from build123d import *

# Parameters (mm, degrees)
SKETCH_1_R          = 6
EXTRUDE_2_DEPTH     = 7.5
CUT_EXTRUDE_START   = -7.5
SKETCH_4_R          = 22.5
CUT_EXTRUDE_4_DEPTH = 2
CUT_EXTRUDE_START_2 = 7.5
SKETCH_4_2_R        = 22.5
CUT_EXTRUDE_5_DEPTH = 2


with BuildPart() as part:
    # 草圖1 → 填料-伸長2 (new body, symmetric)
    with BuildSketch(Plane.XY):
        with BuildLine():
            Line((10.8, 27.988569095), (54.32, 11.195427638))
            ThreePointArc((54.32, 11.195427638), (62, 0), (54.32, -11.195427638))
            Line((54.32, -11.195427638), (10.8, -27.988569095))
            ThreePointArc((10.8, -27.988569095), (2.81349952, -29.867778968), (-5.383437031, -29.513024341))
            ThreePointArc((-5.383437031, -29.513024341), (-23.658051153, -33.253445018), (-34.256327949, -48.603650133))
            ThreePointArc((-34.256327949, -48.603650133), (-47.196522871, -57.898263789), (-57.960436879, -46.151917853))
            ThreePointArc((-57.960436879, -46.151917853), (-46.199430838, -3.114505899), (-13.217722281, 26.931242409))
            ThreePointArc((-13.217722281, 26.931242409), (-1.31940524, 29.97097212), (10.8, 27.988569095))
        make_face()
        with Locations((50, 0)):
            Circle(SKETCH_1_R, mode=Mode.SUBTRACT)
        with Locations((-45.961940777, -45.961940777)):
            Circle(SKETCH_1_R, mode=Mode.SUBTRACT)
        Polygon((15.614971003, -4.18401887), (11.430952133, 11.430952133), (-4.18401887, 15.614971003), (-15.614971003, 4.18401887), (-11.430952133, -11.430952133), (4.18401887, -15.614971003), align=None, mode=Mode.SUBTRACT)
    extrude(amount=EXTRUDE_2_DEPTH, both=True)

    # 草圖4 → 除料-伸長4 (cut)
    with BuildSketch(Plane.XY.offset(CUT_EXTRUDE_START)):
        Circle(SKETCH_4_R)
    extrude(amount=CUT_EXTRUDE_4_DEPTH, mode=Mode.SUBTRACT)

    # 草圖4<2> → 除料-伸長5 (cut)
    with BuildSketch(Plane.XY.offset(CUT_EXTRUDE_START_2)):
        Circle(SKETCH_4_2_R)
    extrude(amount=-CUT_EXTRUDE_5_DEPTH, mode=Mode.SUBTRACT)


solid = part.part
Read the model definition and answer for the solid it produces. Units are mm, in the model's axes. A direction names the side the tool comes from. Coordinates: 2 decimals unless noted, no trailing zeros. Order: outer loops, then holes, each group sorted by start corner. A loop starts at its lowest first (then second) coordinate and runs counter-clockwise, first axis right, second up. Notation, with made-up numbers: (62, -8) - (118, -8) arc R26 cw to (118, 7) - close; hole circle Ø9 at (-36.5, -35). An arc over 180 degrees is marked (long way). Use one line per item in the form item = value.
(1) For a pull along X with two mould halves and no side action, classify faces 1 (the face through (62, 0, 0)), 2 (the face through (44, 0, 0)), 3 (the face through (-1.492, 29.963, 0.105)) as pulls with the +X half, pulls with the -X half, needs draft (parallel to the pull), parting line crosses it, or undercut.
Computed values:
face_1 = pulls with the +X half
face_2 = undercut
face_3 = parting line crosses it
(2) Section B-B, the plane y = 0 is taken. Give the vertices of the cut face in (x, z), then the cut area to 3 significant figures.
Computed values:
outline = (-44.19, -7.5) - (-22.5, -7.5) - (-22.5, -5.5) - (-14.49, -5.5) - (-14.49, 5.5) - (-22.5, 5.5) - (-22.5, 7.5) - (-44.19, 7.5) - close; (14.49, -5.5) - (22.5, -5.5) - (22.5, -7.5) - (44, -7.5) - (44, 7.5) - (22.5, 7.5) - (22.5, 5.5) - (14.49, 5.5) - close; (56, -7.5) - (62, -7.5) - (62, 7.5) - (56, 7.5) - close
area = 914 mm²
(3) Section C-C, the plane z = 2.75 is taken. Give the vertices of the cut face in (x, y).
Computed values:
outline = (-57.96, -46.15) arc R12 ccw to (-34.26, -48.6) arc R25 cw to (-5.38, -29.51) arc R30 ccw to (10.8, -27.99) - (54.32, -11.2) arc R12 ccw to (54.32, 11.2) - (10.8, 27.99) arc R30 ccw to (-13.22, 26.93) arc R80 ccw to start; hole circle Ø12 at (-45.96, -45.96); hole (-15.61, 4.18) - (-11.43, -11.43) - (4.18, -15.61) - (15.61, -4.18) - (11.43, 11.43) - (-4.18, 15.61) - close; hole circle Ø12 at (50, 0)
(4) Which of the six approach directions +Z, -Z, +X, -X, +Y, -Y give full straight-line access (tool end or side, diameter ignored) to faces 4 (the face through (10.382, -19.961, -6.514)), 5 (the face through (10.382, -19.961, 6.514)), 6 (the face through (-13.552, -3.514, 0.077)), 7 (the face through (-23.434, -33.107, 0.105)), 8 (the face through (32.255, 19.71, 0.105))?
Computed values:
face_4 = -Z
face_5 = +Z
face_6 = +Z, -Z
face_7 = +Z, -Z, -Y
face_8 = +Z, -Z, +X, +Y
(5) Section A-A, the plane x = 0 is taken. Give the vertices of the cut face in (y, z), then the cut area to 3 significant figures.
Computed values:
outline = (-30, -7.5) - (-22.5, -7.5) - (-22.5, -5.5) - (-14.49, -5.5) - (-14.49, 5.5) - (-22.5, 5.5) - (-22.5, 7.5) - (-30, 7.5) - close; (14.49, -5.5) - (22.5, -5.5) - (22.5, -7.5) - (30, -7.5) - (30, 7.5) - (22.5, 7.5) - (22.5, 5.5) - (14.49, 5.5) - close
area = 401 mm²
(6) Section D-D, the plane x = 19 is taken. Give the vertices of the cut face in (y, z).
Computed values:
outline = (-24.82, -7.5) - (-12.05, -7.5) - (-12.05, -5.5) - (12.05, -5.5) - (12.05, -7.5) - (24.82, -7.5) - (24.82, 7.5) - (12.05, 7.5) - (12.05, 5.5) - (-12.05, 5.5) - (-12.05, 7.5) - (-24.82, 7.5) - close
(7) Straight lines are drawn through the part: L1, parallel to Y at x = 0, z = 6.5; L2, parallel to Z at x = -19, y = -9; L3, parallel to Y at x = -41.5, z = 1.75. For each, find the intervals that lie inside material, in ascending order.
Computed values:
L1 = -30 to -22.5, 22.5 to 30
L2 = -5.5 to 5.5
L3 = -57.1 to -49.97, -41.95 to 3.74
(8) Given pin 1 Ø1.5 at (x, z) = (8, -0.5) entering from -Y; pin 2 Ø1 at (x, z) = (-7, -5.5) entering from -Y; pin 3 Ø8 at (x, z) = (-2.5, 5.5) entering from -Y, each flat-ended and moving along its own axis, determine where each tip first touches the part or whether it passes through.
Computed values:
pin_1 = -29.11
pin_2 = -29.34
pin_3 = -30
